Design review of the part built by this model. Coordinates are the model's own, in mm. Face numbers are marked on the shaded views. A direction names the side the tool comes from. Round coordinates to 2 decimals unless told otherwise and drop trailing zeros. Use CSV: the item, a comma, the result in double quotes.
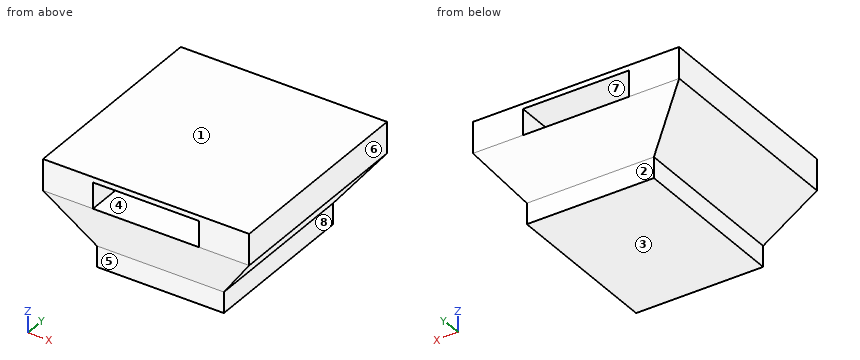
from build123d import *

# Parameters (mm, degrees)
SKETCH030_W           = 12.2
SKETCH030_H           = 15.7
SKETCH031_W           = 12.2
SKETCH031_H           = 15.7
SKETCH032_W           = 19.8
SKETCH032_H           = 19.8
SKETCH033_W           = 19.8
SKETCH033_H           = 19.8
SKETCH034_W           = 10.2
SKETCH034_H           = 15.2
POCKET018_DEPTH       = 2.5
POLARPATTERN003_COUNT = 2


with BuildPart() as part:
    # Sketch030 → AdditiveLoft section 0
    with BuildSketch(Plane.XY):
        Rectangle(SKETCH030_W, SKETCH030_H)
    # Sketch031 → AdditiveLoft section 1
    with BuildSketch(Plane.XY.offset(2)):
        Rectangle(SKETCH031_W, SKETCH031_H)
    # Sketch032 → AdditiveLoft section 2
    with BuildSketch(Plane.XY.offset(7)):
        Rectangle(SKETCH032_W, SKETCH032_H)
    # Sketch033 → AdditiveLoft section 3
    with BuildSketch(Plane.XY.offset(10)):
        Rectangle(SKETCH033_W, SKETCH033_H)
    loft(ruled=True)

    # Sketch034 → Pocket018 (cut)
    with BuildSketch(Plane.XY.offset(9.5)):
        with Locations((0, -11.5)):
            Rectangle(SKETCH034_W, SKETCH034_H)
    pocket018 = extrude(amount=-POCKET018_DEPTH, mode=Mode.SUBTRACT)

    # PolarPattern003: Pocket018 ×2 about axis
    polarpattern003_axis = Axis((0, 0, 9.5), (0, 0, 1))
    for i in range(1, POLARPATTERN003_COUNT):
        add(pocket018.rotate(polarpattern003_axis, i * 360 / POLARPATTERN003_COUNT), mode=Mode.SUBTRACT)


solid = part.part
1) The part is to be moulded in two halves that separate along Z. For the marked faces 1, 2, 3 and 4, say which applies: released by +Z, released by -Z, zero draft, split by the parting line, or undercut.
Answers:
face 1,"released by +Z"
face 2,"zero draft"
face 3,"released by -Z"
face 4,"undercut"
2) Wall thickness on line 1 along X through (y, z) = (5, 9); line 2 along Z through (x, y) = (0.25, -5.25); line 3 along X through (y, z) = (-5.5, 0.75): over which ranges is each line inside the solid? List them lowest first. Write a range as [from, to].
Answers:
line 1,"[-9.9, -5.1], [5.1, 9.9]"
line 2,"[0, 7], [9.5, 10]"
line 3,"[-6.1, 6.1]"
3) For pin 1 Ø2 at (y, z) = (-3.5, 1.5) entering from -X; pin 2 Ø0.6 at (x, z) = (1, 0.5) entering from +Y; pin 3 Ø1.6 at (x, z) = (0, 0.5) entering from -Y, all flat-tipped, find the tip position at first contact; note any pin that passes through.
Answers:
pin 1,"x = -6.48"
pin 2,"y = 7.85"
pin 3,"y = -7.85"
4) Machinability: for the marked faces 5, 6, 7 and 8, which of the approach directions +Z, -Z, +X, -X, +Y, -Y give a long, thin tool a straight path to every point of the face, cutting with its end or side? Answer none if there is none.
Answers:
face 5,"-Z, +X, -X, -Y"
face 6,"+Z, -Z, +X, +Y, -Y"
face 7,"+Y"
face 8,"-Z, +X, +Y, -Y"
